```python
from build123d import *

# Parameters (mm, degrees)
SKETCH_1_R             = 7
SKETCH_1_R_2           = 1.55
EXTRUDE_1_DEPTH        = 2
FILLET_1_R             = 1
CUT_EXTRUDE_START      = -5
CUT_EXTRUDE_1_DEPTH    = 6
FILLET_2_R             = 1
FILLET_2_OF_MIRROR_1_R = 1
SKETCH_3_R             = 1.55
EXTRUDE_2_DEPTH        = 4
FILLET_3_R             = 1
CUT_EXTRUDE_2_DEPTH    = 5
FILLET_4_R             = 1
CUT_EXTRUDE_3_DEPTH    = 5
EXTRUDE_3_DEPTH        = 4
SKETCH_8_R             = 0.75
CUT_EXTRUDE_4_DEPTH    = 5
FILLET_5_R             = 1.5
CUT_EXTRUDE_5_DEPTH    = 5
EXTRUDE_4_DEPTH        = 4
CUT_EXTRUDE_6_DEPTH    = 5
SKETCH_12_R            = 1
CUT_EXTRUDE_7_DEPTH    = 5
FILLET_6_R             = 3
FILLET_7_R             = 1
FILLET_8_R             = 1


with BuildPart() as part:
    # 草图1 → 凸台-拉伸1 (new body, symmetric)
    with BuildSketch(Plane.XY):
        with BuildLine():
            Line((-17.5, 11), (-10, 11))
            Line((-10, 11), (-8.321800738, 9))
            Line((-8.321800738, 9), (8.321800738, 9))
            Line((8.321800738, 9), (10, 11))
            Line((10, 11), (17.5, 11))
            ThreePointArc((17.5, 11), (17.577641076, 10.999138732), (17.655243941, 10.99655535))
            Line((17.655243941, 10.99655535), (37, 10.137665421))
            Line((37, 10.137665421), (28.942548731, -12))
            Line((28.942548731, -12), (17.199216279, -10.987051642))
            ThreePointArc((17.199216279, -10.987051642), (15.184578245, -10.124656567), (14.077678472, -8.233290774))
            Line((14.077678472, -8.233290774), (2.304628146, -10.75586766))
            ThreePointArc((2.304628146, -10.75586766), (0, -11), (-2.304628146, -10.75586766))
            Line((-2.304628146, -10.75586766), (-14.077678472, -8.233290774))
            ThreePointArc((-14.077678472, -8.233290774), (-15.184578245, -10.124656567), (-17.199216279, -10.987051642))
            Line((-17.199216279, -10.987051642), (-28.942548731, -12))
            Line((-28.942548731, -12), (-37, 10.137665421))
            Line((-37, 10.137665421), (-17.655243941, 10.99655535))
            ThreePointArc((-17.655243941, 10.99655535), (-17.577641076, 10.999138732), (-17.5, 11))
        make_face()
        Circle(SKETCH_1_R, mode=Mode.SUBTRACT)
        with Locations((17.5, 7.5)):
            Circle(SKETCH_1_R_2, mode=Mode.SUBTRACT)
        with Locations((17.5, -7.5)):
            Circle(SKETCH_1_R_2, mode=Mode.SUBTRACT)
        with Locations((-17.5, -7.5)):
            Circle(SKETCH_1_R_2, mode=Mode.SUBTRACT)
        with Locations((-17.5, 7.5)):
            Circle(SKETCH_1_R_2, mode=Mode.SUBTRACT)
    extrude(amount=EXTRUDE_1_DEPTH, both=True)

    # 圆角1
    fillet_1_edges = [part.edges().sort_by_distance(p)[0] for p in [
        (14.077678472, -8.233290774, 0),
        (-14.077678472, -8.233290774, 0),
    ]]
    fillet(fillet_1_edges, radius=FILLET_1_R)

    # 草图2 → 切除-拉伸1 (cut)
    with BuildSketch(Plane.XY.offset(2).offset(CUT_EXTRUDE_START)):
        Polygon((-20.5, 7.867295251), (-32.782632739, 7.321957304), (-27.222903771, -7.953272497), align=None)
        with BuildLine():
            Line((-19.251811465, 4.412338006), (-24.573190843, -8.11011447))
            Line((-24.573190843, -8.11011447), (-21.036866665, -7.805080632))
            ThreePointArc((-21.036866665, -7.805080632), (-20.623106229, -5.812188553), (-19.182687898, -4.374130291))
            Line((-19.182687898, -4.374130291), (-15.331076504, 4.689613751))
            ThreePointArc((-15.331076504, 4.689613751), (-17.24956823, 3.958844267), (-19.251811465, 4.412338006))
        make_face()
    cut_extrude_1 = extrude(amount=CUT_EXTRUDE_1_DEPTH, mode=Mode.SUBTRACT)

    # 圆角2
    fillet_2_edges = [part.edges().sort_by_distance(p)[0] for p in [
        (-20.5, 7.867295251, 0),
        (-27.222903771, -7.953272497, 0),
        (-32.782632739, 7.321957304, 0),
        (-19.251811465, 4.412338006, 0),
        (-15.331076504, 4.689613751, 0),
        (-19.182687898, -4.374130291, 0),
        (-21.036866665, -7.805080632, 0),
        (-24.573190843, -8.11011447, 0),
    ]]
    fillet(fillet_2_edges, radius=FILLET_2_R)

    # 镜向1: 切除-拉伸1 across plane
    add(cut_extrude_1.mirror(Plane(origin=(0, 0, 0), x_dir=(0, 0, 1), z_dir=(1, 0, 0))), mode=Mode.SUBTRACT)

    # 圆角2 of 镜向1
    fillet_2_of_mirror_1_edges = [part.edges().sort_by_distance(p)[0] for p in [
        (20.5, 7.867295251, 0),
        (27.222903771, -7.953272497, 0),
        (32.782632739, 7.321957304, 0),
        (19.251811465, 4.412338006, 0),
        (15.331076504, 4.689613751, 0),
        (19.182687898, -4.374130291, 0),
        (21.036866665, -7.805080632, 0),
        (24.573190843, -8.11011447, 0),
    ]]
    fillet(fillet_2_of_mirror_1_edges, radius=FILLET_2_OF_MIRROR_1_R)

    # 草图3 → 凸台-拉伸2 (add)
    with BuildSketch(Plane.XY.offset(2)):
        with BuildLine():
            Line((-37.69913918, 12.058534531), (-37, 10.137665421))
            Line((-37, 10.137665421), (-32.4761474, 10.338520445))
            ThreePointArc((-32.4761474, 10.338520445), (-33.315445081, 16.579981486), (-37.69913918, 12.058534531))
        make_face()
        with Locations((-34.410215007, 13.255605032)):
            Circle(SKETCH_3_R, mode=Mode.SUBTRACT)
        with BuildLine():
            Line((-27.557621455, -15.805056417), (-28.942548731, -12))
            Line((-28.942548731, -12), (-22.730405687, -11.464157204))
            ThreePointArc((-22.730405687, -11.464157204), (-21.928391725, -17.210478932), (-27.557621455, -15.805056417))
        make_face()
        with Locations((-24.268697282, -14.607985915)):
            Circle(SKETCH_3_R, mode=Mode.SUBTRACT)
    extrude_2 = extrude(amount=-EXTRUDE_2_DEPTH)

    # 镜向2: 凸台-拉伸2 across plane
    add(extrude_2.mirror(Plane(origin=(0, 0, 0), x_dir=(0, 0, 1), z_dir=(1, 0, 0))))

    # 圆角3
    fillet_3_edges = [part.edges().sort_by_distance(p)[0] for p in [
        (-22.730405687, -11.464157204, 0),
        (-32.4761474, 10.338520445, 0),
        (22.730405687, -11.464157204, 0),
        (32.4761474, 10.338520445, 0),
    ]]
    fillet(fillet_3_edges, radius=FILLET_3_R)

    # 草图4 → 切除-拉伸2 (cut, through all)
    with BuildSketch(Plane.XY.offset(2)):
        with BuildLine():
            Line((-16.384851826, -4.1824038), (-12.057869255, 6))
            Line((-12.057869255, 6), (-8, 6))
            ThreePointArc((-8, 6), (-9.993390733, -0.363512948), (-7.542930102, -6.565379309))
            Line((-7.542930102, -6.565379309), (-15.108699944, -4.944284045))
            ThreePointArc((-15.108699944, -4.944284045), (-15.705867849, -4.49482283), (-16.384851826, -4.1824038))
        make_face()
    cut_extrude_2 = extrude(amount=-CUT_EXTRUDE_2_DEPTH, mode=Mode.SUBTRACT)

    # 镜向3: 切除-拉伸2 across plane
    add(cut_extrude_2.mirror(Plane(origin=(0, 0, 0), x_dir=(0, 0, 1), z_dir=(1, 0, 0))), mode=Mode.SUBTRACT)

    # 圆角4
    fillet_4_edges = [part.edges().sort_by_distance(p)[0] for p in [
        (-12.057869255, 6, 0),
        (-8, 6, 0),
        (-7.542930102, -6.565379309, 0),
        (-15.108699944, -4.944284045, 0),
        (-16.384851826, -4.1824038, 0),
        (8, 6, 0),
        (12.057869255, 6, 0),
        (16.384851826, -4.1824038, 0),
        (15.108699944, -4.944284045, 0),
        (7.542930102, -6.565379309, 0),
    ]]
    fillet(fillet_4_edges, radius=FILLET_4_R)

    # 草图5 → 切除-拉伸3 (cut, through all)
    with BuildSketch(Plane.XY.offset(2)):
        Polygon((30.884976598, -6.370842854), (33.798023723, -7.431105298), (37.25242717, 2.059790172), (34.339380046, 3.120052616), align=None)
    cut_extrude_3 = extrude(amount=-CUT_EXTRUDE_3_DEPTH, mode=Mode.SUBTRACT)

    # 草图7 → 凸台-拉伸3 (add)
    with BuildSketch(Plane.XY.offset(2)):
        Polygon((35.271298659, 5.388097522), (40.439608074, 3.506986734), (35.309305924, -10.588402578), (30.140996509, -8.707291789), (30.97894586, -6.405044868), (33.798023723, -7.431105298), (37.25242717, 2.059790172), (34.433349308, 3.085850601), align=None)
    extrude_3 = extrude(amount=-EXTRUDE_3_DEPTH)

    # 镜向4: 切除-拉伸3, 凸台-拉伸3 across plane
    add(cut_extrude_3.mirror(Plane(origin=(0, 0, 0), x_dir=(0, 0, 1), z_dir=(1, 0, 0))), mode=Mode.SUBTRACT)
    add(extrude_3.mirror(Plane(origin=(0, 0, 0), x_dir=(0, 0, 1), z_dir=(1, 0, 0))))

    # 草图8 → 切除-拉伸4 (cut, through all)
    with BuildSketch(Plane(origin=(0, 0, -2), x_dir=(-1, 0, 0), z_dir=(0, 0, -1))):
        with Locations((-36.995912063, 1.355020706)):
            Circle(SKETCH_8_R)
        with Locations((-34.082864939, 2.41528315)):
            Circle(SKETCH_8_R)
        with Locations((-34.05453883, -6.726335833)):
            Circle(SKETCH_8_R)
        with Locations((-31.141491706, -5.666073389)):
            Circle(SKETCH_8_R)
        with Locations((-35.527813767, 6.092866988)):
            Circle(SKETCH_8_R)
        with Locations((-29.884481402, -9.412061255)):
            Circle(SKETCH_8_R)
    cut_extrude_4 = extrude(amount=-CUT_EXTRUDE_4_DEPTH, mode=Mode.SUBTRACT)

    # 镜向5: 切除-拉伸4 across plane
    add(cut_extrude_4.mirror(Plane(origin=(0, 0, 0), x_dir=(0, 0, 1), z_dir=(1, 0, 0))), mode=Mode.SUBTRACT)

    # 圆角5
    fillet_5_edges = [part.edges().sort_by_distance(p)[0] for p in [
        (40.439608074, 3.506986734, 0),
        (35.309305924, -10.588402578, 0),
        (-40.439608074, 3.506986734, 0),
        (-35.309305924, -10.588402578, 0),
    ]]
    fillet(fillet_5_edges, radius=FILLET_5_R)

    # 草图9 → 切除-拉伸5 (cut, through all)
    with BuildSketch(Plane(origin=(0, 0, -2), x_dir=(-1, 0, 0), z_dir=(0, 0, -1))):
        with BuildLine():
            Line((-32.316536273, 6.041367788), (-33.695268787, 9.829404235))
            ThreePointArc((-33.695268787, 9.829404235), (-30.928713694, 13.614977548), (-34.410215007, 16.755605032))
            Line((-34.410215007, 16.755605032), (45.589784993, 16.755605032))
            Line((45.589784993, 16.755605032), (45.589784993, -18.107985915))
            Line((45.589784993, -18.107985915), (-24.268697282, -18.107985915))
            ThreePointArc((-24.268697282, -18.107985915), (-20.874243549, -13.754942039), (-25.923336124, -11.523805262))
            Line((-25.923336124, -11.523805262), (-28.090663396, -5.56912252))
            Line((-28.090663396, -5.56912252), (-32.316536273, 6.041367788))
        make_face()
    extrude(amount=-CUT_EXTRUDE_5_DEPTH, mode=Mode.SUBTRACT)

    # 草图10 → 凸台-拉伸4 (add)
    with BuildSketch(Plane(origin=(0, 0, -2), x_dir=(-1, 0, 0), z_dir=(0, 0, -1))):
        with BuildLine():
            Line((-32.323351951, 10.445800309), (-24.476175097, -11.114140905))
            ThreePointArc((-24.476175097, -11.114140905), (-25.222020853, -11.240319933), (-25.923336124, -11.523805262))
            Line((-25.923336124, -11.523805262), (-33.695268787, 9.829404235))
            ThreePointArc((-33.695268787, 9.829404235), (-32.975809264, 10.063038641), (-32.323351951, 10.445800309))
        make_face()
    extrude(amount=-EXTRUDE_4_DEPTH)

    # 草图11 → 切除-拉伸6 (cut, through all)
    with BuildSketch(Plane(origin=(0, 0, -2), x_dir=(-1, 0, 0), z_dir=(0, 0, -1))):
        Polygon((-30.016621436, 4.108110305), (-30.995676903, 2.412336493), (-28.778462541, -3.6794099), (-26.938440146, -4.349123282), align=None)
    extrude(amount=-CUT_EXTRUDE_6_DEPTH, mode=Mode.SUBTRACT)

    # 草图12 → 切除-拉伸7 (cut, through all)
    with BuildSketch(Plane(origin=(0, 0, -2), x_dir=(-1, 0, 0), z_dir=(0, 0, -1))):
        with Locations((-31.981331808, 9.506107688)):
            Circle(SKETCH_12_R)
        with Locations((-24.81819524, -10.174448284)):
            Circle(SKETCH_12_R)
    extrude(amount=-CUT_EXTRUDE_7_DEPTH, mode=Mode.SUBTRACT)

    # 圆角6
    fillet_6_edges = [part.edges().sort_by_distance(p)[0] for p in [
        (24.476175097, -11.114140905, 0),
        (32.323351951, 10.445800309, 0),
    ]]
    fillet(fillet_6_edges, radius=FILLET_6_R)

    # 圆角7
    fillet_7_edges = [part.edges().sort_by_distance(p)[0] for p in [
        (28.778462541, -3.6794099, 0),
        (30.995676903, 2.412336493, 0),
    ]]
    fillet(fillet_7_edges, radius=FILLET_7_R)

    # 圆角8
    fillet_8_edges = [part.edges().sort_by_distance(p)[0] for p in [
        (30.016621436, 4.108110305, 0),
        (26.938440146, -4.349123282, 0),
        (31.639311664, 8.566415067, 0),
        (25.160215383, -9.234755664, 0),
    ]]
    fillet(fillet_8_edges, radius=FILLET_8_R)


solid = part.part
```
Model file for the job. Use its own axes, mm. A direction names the side the tool comes from. Round coordinates to 2 decimals unless told otherwise and drop trailing zeros. Write each loop counter-clockwise with the first axis right and the second up, starting at its lowest first coordinate (ties: lowest second). Pieces come first, ordered by that corner, then holes. Notation, with made-up numbers: (-38.75, -20.5) - (-31.75, -20.5) arc R21 ccw to (-31.75, 3.5) - close; hole circle Ø4 at (-1, -34). An arc over 180 degrees is marked (long way). Use CSV: the item, a comma, the result in double quotes. Start each with the question number.
Item 1: Band-saw the part on C-C (z = -1.65). State how many separate pieces and enclosed holes the cut face has, and give its area (3 significant figures).
Item 2: Band-saw the part on B-B (y = -5.5). Write the cut outline in (x, z), and give its area (3 significant figures).
Item 3: Band-saw the part on D-D (x = 38.5). Write the cut outline in (y, z), and give its area (3 significant figures).
Item 4: Band-saw the part on A-A (y = 1). Write the cut outline in (x, z), and give its area (3 significant figures).
Item 5: Tool access for faces 1 (the face through (32.63, -1.58, 0.03)), 2 (the face through (29.9, -0.6, 0)), 3 (the face through (35.1, -10, 0)): list every direction of +Z, -Z, +X, -X, +Y, -Y with a clear straight run to the whole face (end or side of a thin tool).
Item 6: Two-plate mould, pull along Y, no slides. Class faces 4 (the face through (27.9, -4, 0)), 5 (the face through (34.818, 6.334, -0.028)), 6 (the face through (35.51, -2.73, 0.03)), 7 (the face through (32.05, -9.4, 0.03)): released by +Y, released by -Y, zero draft, split by the parting line, or undercut.
Item 7: Pin check, flat tip, straight feed: P1, Ø1, axis at x = 32.5, z = -0.5, coming from the +Y side. Stop position of the tip, or through.
Item 8: Drill centre lines: L1, parallel to Y at x = 34, z = -1.15; L2, parallel to X at y = -14, z = 0.25; L3, parallel to X at y = 1, z = 0.75. Where is each one in solid material? Low to high. Write a range as [from, to].
Checked values:
1,separate pieces,"1"
1,enclosed holes,"3"
1,area,"199 mm²"
2,outline,"(26.52, -2) - (30.41, -2) - (30.41, 2) - (26.52, 2) - close; (34.5, -2) - (37.16, -2) - (37.16, 2) - (34.5, 2) - close"
2,area,"26.2 mm²"
3,outline,"(-1.82, -2) - (4.21, -2) - (4.21, 2) - (-1.82, 2) - close"
3,area,"24.1 mm²"
4,outline,"(30.48, -2) - (33.57, -2) - (33.57, 2) - (30.48, 2) - close; (37.66, -2) - (39.53, -2) - (39.53, 2) - (37.66, 2) - close"
4,area,"19.8 mm²"
5,face 1,"+Z, -Z"
5,face 2,"+Z, -Z, -X"
5,face 3,"+Z, -Z, -Y"
6,face 4,"released by +Y"
6,face 5,"undercut"
6,face 6,"undercut"
6,face 7,"released by -Y"
7,P1,"stops at y = 16.46"
8,L1,"y = [-10.11, -7.47], [3.16, 11.76], [14.75, 16.73]"
8,L2,"x = [20.82, 22.84], [25.69, 28.21]"
8,L3,"x = [30.48, 33.57], [37.66, 39.53]"
